Could you check a few things on this model? Use its own coordinates, in mm. A direction names the side the tool comes from. Coordinates: 2 decimals unless noted, no trailing zeros. Order: outer loops, then holes, each group sorted by start corner. A loop starts at its lowest first (then second) coordinate and runs counter-clockwise, first axis right, second up. Notation, with made-up numbers: (80, 19) -> (99, 19) arc R14 ccw to (99, 46) -> close; hole circle Ø1 at (-13, 67). An arc over 180 degrees is marked (long way). Use a Markdown table: item, result. Add a question column.
1) If we section it at C-C (y = 9.75): Write out the boundary of the cut face in (x, z).
2) Will these pins go through, and if not, where does the flat tip stop? pin 1 Ø3.5 at (y, z) = (3, 5.5) entering from +X; pin 2 Ø5 at (x, z) = (11, 2.5) entering from -Y.
3) If we section it at D-D (z = 1): Write out the boundary of the cut face in (x, y), plus the area to 3 significant figures.
4) If I drill on L1, parallel to X at y = 11, z = 3.75; L2, parallel to Y at x = 6.5, z = 5.25; L3, parallel to Y at x = 1.25, z = 1.25, over which ranges is the centre line in solid material (lowest first)? Write a range as [from, to].
5) Which directions (+Z, -Z, +X, -X, +Y, -Y) give clear straight access to the entire face, cutting with the end or side of a thin tool? Please do faces 1 (the flat face through (11, 11.3, 6)), 2 (the flat face through (9, 25.4, 5)).
6) If we section it at B-B (z = 8.5): Write out the boundary of the cut face in (x, y).
7) If we section it at A-A (x = 6.5): Write out the boundary of the cut face in (y, z).
```python
from build123d import *

# Parameters (mm, degrees)
F0_W     = 16.4
F0_H     = 25.4
F1_DEPTH = 11.3
F2_W     = 11.3
F2_H     = 11.3
F3_DEPTH = 25
F4_R     = 2
F5_R     = 1


with BuildPart() as f1:
    # F0 (on Top) → F1 (new body)
    with BuildSketch(Plane.XY):
        with Locations((8.2, 12.7)):
            Rectangle(F0_W, F0_H)
    extrude(amount=F1_DEPTH)

    # F2 (on face) → F3 (cut)
    with BuildSketch(Plane.XY.offset(11.3)):
        with Locations((10.75, 5.65)):
            Rectangle(F2_W, F2_H)
    extrude(amount=-F3_DEPTH, mode=Mode.SUBTRACT)

    # F4
    f4_edges = [f1.edges().sort_by_distance(p)[0] for p in [
        (16.4, 18.35, 0),
        (2.55, 0, 0),
    ]]
    fillet(f4_edges, radius=F4_R)

    # F5
    f5_edges = [f1.edges().sort_by_distance(p)[0] for p in [
        (0, 25.4, 5.65),
        (0, 12.7, 11.3),
        (8.2, 25.4, 11.3),
    ]]
    fillet(f5_edges, radius=F5_R)


solid = f1.part
```
Answer sheet:
| question | item | result |
|---|---|---|
| 1 | outline | (0, 0) -> (5.1, 0) -> (5.1, 11.3) -> (1, 11.3) arc R1 ccw to (0, 10.3) -> close |
| 2 | pin 1 | x = 5.1 |
| 2 | pin 2 | y = 11.3 |
| 3 | outline | (0, 0.27) -> (5.1, 0.27) -> (5.1, 11.3) -> (16.13, 11.3) -> (16.13, 25.4) -> (1, 25.4) arc R1 ccw to (0, 24.4) -> close |
| 3 | area | 284 mm2 |
| 4 | L1 | [0, 5.1] |
| 4 | L2 | [11.3, 25.4] |
| 4 | L3 | [0.15, 25.4] |
| 5 | face 1 | +Z, -Z, +X, -Y |
| 5 | face 2 | +Z, -Z, +X, -X, +Y |
| 6 | outline | (0, 0) -> (5.1, 0) -> (5.1, 11.3) -> (16.4, 11.3) -> (16.4, 25.4) -> (1, 25.4) arc R1 ccw to (0, 24.4) -> close |
| 7 | outline | (11.3, 0) -> (25.4, 0) -> (25.4, 10.3) arc R1 ccw to (24.4, 11.3) -> (11.3, 11.3) -> close |
